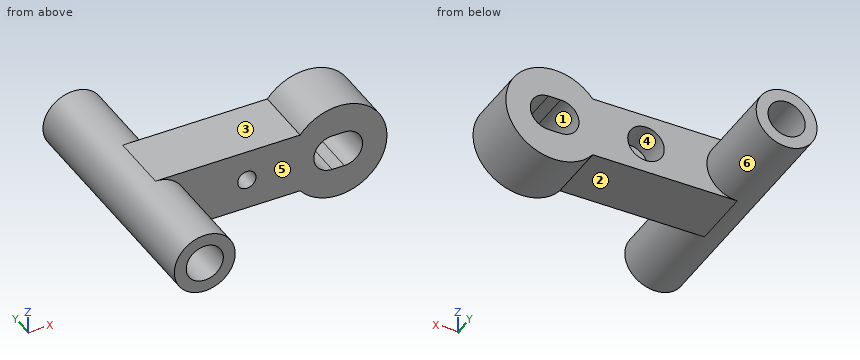
from build123d import *

# Parameters (mm, degrees)
SKETCH008_R     = 3.05
SKETCH008_R_2   = 1.5
PAD003_DEPTH    = 5
SKETCH009_R     = 5
SKETCH009_R_2   = 3.05
PAD004_DEPTH    = 20
SKETCH011_R     = 3
POCKET004_DEPTH = 10


with BuildPart() as part:
    # Sketch008 → Pad003 (new body, symmetric)
    with BuildSketch(Plane.XZ):
        with BuildLine():
            ThreePointArc((-15, 5), (-20, 0), (-15, -5))
            Line((-15, -5), (8.746454, -5))
            ThreePointArc((8.746454, -5), (23.006674, 0), (8.746454, 5))
            Line((-15, 5), (8.746454, 5))
        make_face()
        with Locations((-15, 0)):
            Circle(SKETCH008_R, mode=Mode.SUBTRACT)
        Circle(SKETCH008_R_2, mode=Mode.SUBTRACT)
        with BuildLine():
            ThreePointArc((14, 3), (11, 0), (14, -3))
            Line((14, -3), (16, -3))
            ThreePointArc((16, -3), (19, 0), (16, 3))
            Line((14, 3), (16, 3))
        make_face(mode=Mode.SUBTRACT)
    extrude(amount=PAD003_DEPTH, both=True)

    # Sketch009 → Pad004 (join, symmetric)
    with BuildSketch(Plane.XZ):
        with Locations((-15, 0)):
            Circle(SKETCH009_R)
        with Locations((-15, 0)):
            Circle(SKETCH009_R_2, mode=Mode.SUBTRACT)
    extrude(amount=PAD004_DEPTH, both=True)

    # Sketch011 → Pocket004 (cut)
    with BuildSketch(Plane.XZ):
        Circle(SKETCH011_R)
    extrude(amount=-POCKET004_DEPTH, mode=Mode.SUBTRACT)


with BuildPart() as part_1:
    # Body017 placement: moved
    add(part.part.moved(Location((0, 40.5, 0))))


solid = part_1.part
Source: CAD feature listing. Evaluate the final solid. Frame: model axes, mm. Face numbers are marked on the shaded views. A direction names the side the tool comes from. Give positions to 0.01 mm unless a question says otherwise; leave off trailing zeros. Write each loop counter-clockwise with the first axis right and the second up, starting at its lowest first coordinate (ties: lowest second). Pieces come first, ordered by that corner, then holes. Notation, with made-up numbers: M 25,23 L 34,23 A11 cw 34,35 Z; hole C 13,-26 d9. An arc over 180 degrees is marked long. Answer as a JSON object with one key per item and string values.
Q1. Mould query, pull axis X, two halves, no side actions, for the marked faces 4, 5 and 6. Classes: +X half, -X half, draft (parallel to the pull), parting line (faces both ways), or undercut.
Geometry check:
{"face 4": "undercut", "face 5": "draft", "face 6": "parting line"}
Q2. Cut plane A-A, the plane x = 15. Return the cut outline in (y, z), then the cut area to 3 significant figures.
Geometry check:
{"outline": "M 35.5,-8.01 L 45.5,-8.01 L 45.5,-3 L 35.5,-3 Z; M 35.5,3 L 45.5,3 L 45.5,8.01 L 35.5,8.01 Z", "area": "100 mm^2"}
Q3. Cut plane D-D, the plane x = 0. Return the cut outline in (y, z), then the cut area to 3 significant figures.
Geometry check:
{"outline": "M 35.5,-5 L 45.5,-5 L 45.5,-3 L 40.5,-3 L 40.5,-1.5 L 35.5,-1.5 Z; M 35.5,1.5 L 40.5,1.5 L 40.5,3 L 45.5,3 L 45.5,5 L 35.5,5 Z", "area": "55.0 mm^2"}
Q4. Cut plane C-C, the plane y = 26. Return the cut outline in (x, z).
Geometry check:
{"outline": "C -15,0 d10; hole C -15,0 d6.1"}
Q5. Ray query, line 1 along X through (y, z) = (31.5, 0.25); line 2 along Z through (x, y) = (-15, 31); line 3 along X through (y, z) = (43, 2). Return the intervals inside material, ascending.
Geometry check:
{"line 1": "x = -19.99 to -18.04, -11.96 to -10.01", "line 2": "z = -5 to -3.05, 3.05 to 5", "line 3": "x = -19.58 to -17.3, -12.7 to -2.24, 2.24 to 11.76, 18.24 to 22.75"}
Q6. Access query for the marked faces 1, 2 and 3. Directions: +Z, -Z, +X, -X, +Y, -Y. A direction counts if a zero-diameter tool reaches every point of the face in a straight line with its end or side. Return the directions, or none.
Geometry check:
{"face 1": "+Y, -Y", "face 2": "-Z, -X, +Y, -Y", "face 3": "+Z, -X, +Y, -Y"}
Q7. Cut plane B-B, the plane z = 0. Return the cut outline in (x, y).
Geometry check:
{"outline": "M -20,20.5 L -18.05,20.5 L -18.05,60.5 L -20,60.5 Z; M -11.95,20.5 L -10,20.5 L -10,35.5 L -1.5,35.5 L -1.5,40.5 L -3,40.5 L -3,45.5 L -10,45.5 L -10,60.5 L -11.95,60.5 Z; M 1.5,35.5 L 11,35.5 L 11,45.5 L 3,45.5 L 3,40.5 L 1.5,40.5 Z; M 19,35.5 L 23.01,35.5 L 23.01,45.5 L 19,45.5 Z"}
Q8. Contact query for flat-ended pins moving along their axis: P1, Ø1, axis at x = 3.5, z = 3.5, coming from the +Y side; P2, Ø3, axis at x = 11.5, y = 44.5, coming from the -Z side; P3, Ø3, axis at x = 18.5, z = -4, coming from the -Y side. Output: stop coordinate, or through.
Geometry check:
{"P1": "stops at y = 45.5", "P2": "stops at z = -7.75", "P3": "stops at y = 35.5"}
